```python
from build123d import *

# Parameters (mm, degrees)
BASPROSKE_W     = 2
BASPROSKE_H     = 16
TOOTHCUT_DEPTH  = 23.715633383
TEETHCUTS_COUNT = 30
BORSKE_R        = 6
BORE_DEPTH      = 50.0000508


with BuildPart() as part:
    # BasProSke → Base-Revolve (revolve)
    with BuildSketch(Plane(origin=(0, 0, 0), x_dir=(1, 0, 0), z_dir=(0, 1, 0)), mode=Mode.PRIVATE) as base_revolve_sk:
        with Locations((1, 8)):
            Rectangle(BASPROSKE_W, BASPROSKE_H)
    revolve(base_revolve_sk.sketch.rotate(Axis((-10, 0, 0), (1, 0, 0)), 180), axis=Axis((-10, 0, 0), (1, 0, 0)))

    # TooCutSke → ToothCut (cut, through all)
    with BuildSketch(Plane(origin=(0, 0, 0), x_dir=(0, 0, -1), z_dir=(1, 0, 0))):
        with BuildLine():
            ThreePointArc((0.466400716, 13.741086979), (0, 13.749), (-0.466400716, 13.741086979))
            ThreePointArc((-0.466400716, 13.741086979), (-0.819142092, 14.899954875), (-1.3974676, 15.964351834))
            ThreePointArc((-1.3974676, 15.964351834), (0, 16.0254), (1.3974676, 15.964351834))
            ThreePointArc((1.3974676, 15.964351834), (0.819142092, 14.899954875), (0.466400716, 13.741086979))
        make_face()
    toothcut = extrude(amount=TOOTHCUT_DEPTH, mode=Mode.SUBTRACT)

    # TeethCuts: ToothCut ×30 about axis
    teethcuts_axis = Axis((0, 0, 0), (1, 0, 0))
    for i in range(1, TEETHCUTS_COUNT):
        add(toothcut.rotate(teethcuts_axis, i * 360 / TEETHCUTS_COUNT), mode=Mode.SUBTRACT)

    # BorSke → Bore (cut, symmetric)
    with BuildSketch(Plane(origin=(0, 0, 0), x_dir=(0, 0, -1), z_dir=(1, 0, 0))):
        with Locations(Location((0, 0, 0), (0, 0, 180))):
            Circle(BORSKE_R)
    extrude(amount=BORE_DEPTH, both=True, mode=Mode.SUBTRACT)


solid = part.part
```
Input: part model. Units: mm. Frame: model coordinates. A direction names the side the tool comes from. Coordinates: 2 decimals unless noted, no trailing zeros. Write each loop counter-clockwise with the first axis right and the second up, starting at its lowest first coordinate (ties: lowest second). Pieces come first, ordered by that corner, then holes. Notation, with made-up numbers: (10, 83) -> (37, 83) arc R27 ccw to (37, 103) -> close; hole circle Ø3 at (33.25, 51). An arc over 180 degrees is marked (long way). Answer as a JSON object with one key per item and string values.
1. Section A-A on z = 0. Return the cut outline in (x, y).
Result set:
{"outline": "(0, -13.75) -> (2, -13.75) -> (2, -6) -> (0, -6) -> close; (0, 6) -> (2, 6) -> (2, 13.75) -> (0, 13.75) -> close"}
2. First-contact query: P1, Ø3, axis at y = -10.5, z = -6.5, coming from the -X side. Flat tip, straight axial feed; report the tip coordinate or a pass-through.
Result set:
{"P1": "stops at x = 0"}
3. Material intervals for line 1 (Y direction, x = 0.45, z = 0); line 2 (Z direction, x = 1.15, y = 9); line 3 (Z direction, x = 0.1, y = 4), sorted ascending. Write a range as from..to.
Result set:
{"line 1": "y = -13.75..-6, 6..13.75", "line 2": "z = -13.03..-10.79, -10.39..10.39, 10.79..13.03", "line 3": "z = -13.15..-4.47, 4.47..13.15"}
4. Access query for faces 4 (the face through (0.986, -14.378, -3.881)), 5 (the face through (0.986, -6.88, -11.904)), 6 (the face through (0.986, 1.431, -13.674)), 7 (the face through (0.99, 2.37, 14.73)), 8 (the face through (0.99, 13.26, 6.79)). Directions: +Z, -Z, +X, -X, +Y, -Y. A direction counts if a zero-diameter tool reaches every point of the face in a straight line with its end or side. Return the directions, or none.
Result set:
{"face 4": "+X, -X, -Y", "face 5": "+X, -X", "face 6": "-Z, +X, -X", "face 7": "+Z, +X, -X", "face 8": "+X, -X, +Y"}
5. Mould query, pull axis Y, two halves, no side actions, for faces 1 (the face through (0.99, -13.75, 0.01)), 2 (the face through (0.99, 6.87, -11.91)), 3 (the face through (0.986, 14.406, -3.9)). Classes: released by +Y, released by -Y, zero draft, split by the parting line, or undercut.
Result set:
{"face 1": "released by -Y", "face 2": "undercut", "face 3": "released by +Y"}
